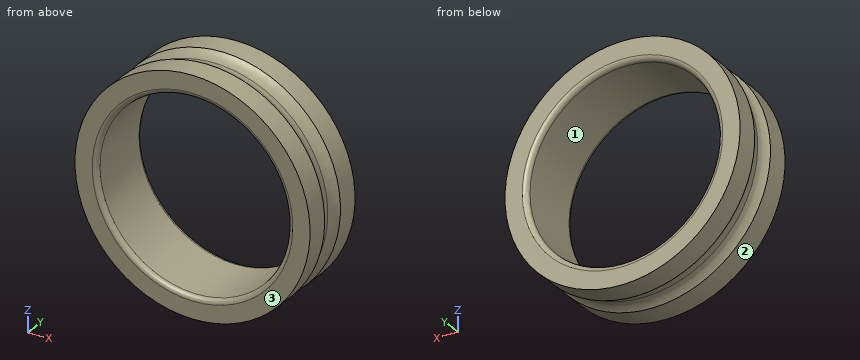
from build123d import *

# Parameters (mm, degrees)
FILLET1_R = 1


with BuildPart() as part:
    # Sketch1 → Revolve2 (revolve)
    with BuildSketch(Plane.XY, mode=Mode.PRIVATE) as revolve2_sk:
        with BuildLine():
            ThreePointArc((-23.61875, 7.5), (-23.878834577, 6.086926278), (-24.625, 4.859058821))
            Line((-24.625, 4.859058821), (-24.625, 0))
            Line((-24.625, 0), (-20, 0))
            Line((-20, 0), (-20, 15))
            Line((-20, 15), (-24.625, 15))
            Line((-24.625, 15), (-24.625, 10.140941179))
            ThreePointArc((-24.625, 10.140941179), (-23.878834577, 8.913073722), (-23.61875, 7.5))
        make_face()
    revolve(revolve2_sk.sketch.rotate(Axis((0, 0, 0), (0, 1, 0)), 270), axis=Axis((0, 0, 0), (0, 1, 0)))

    # Fillet1
    fillet1_edges = [part.edges().sort_by_distance(p)[0] for p in [
        (0, 15, 20),
        (0, 0, 20),
    ]]
    fillet(fillet1_edges, radius=FILLET1_R)


solid = part.part
The listing builds one solid part. Answer for the finished solid, in the listing's coordinates (mm). Face numbers are marked on the shaded views. Round coordinates to 2 decimals unless told otherwise and drop trailing zeros. Order: outer loops, then holes, each group sorted by start corner. A loop starts at its lowest first (then second) coordinate and runs counter-clockwise, first axis right, second up. Notation, with made-up numbers: (27, 48) -> (78, 48) arc R25 ccw to (78, 75) -> close; hole circle Ø7 at (75, 22.5). An arc over 180 degrees is marked (long way). One line per item, written item: value.
Item 1: Given P1, Ø1.5, axis at x = -17.5, y = 9, coming from the -Z side; P2, Ø6, axis at y = 10, z = 18, coming from the +X side; P3, Ø8, axis at x = -6, y = 8.5, coming from the -Z side, each flat-ended and moving along its own axis, determine where each tip first touches the part or whether it passes through.
Taken from the geometry:
P1: stops at z = -17.23
P2: stops at x = 19.53
P3: stops at z = -24.51
Item 2: Find section A-A, the plane y = 2.75. Give the vertices of the cut face in (x, z) (3 decimals), then the cut area to 3 significant figures.
Taken from the geometry:
outline: circle Ø49.25 at (0, 0); hole circle Ø40 at (0, 0)
area: 648 mm2
Item 3: Find section B-B, the plane y = 5.75. Give the vertices of the cut face in (x, z), then the cut area to 3 significant figures.
Taken from the geometry:
outline: circle Ø48.05 at (0, 0); hole circle Ø40 at (0, 0)
area: 557 mm2
Item 4: For a pull along Z with two mould halves and no side action, classify the marked faces 1, 2 and 3 as released by +Z, released by -Z, zero draft, split by the parting line, or undercut.
Taken from the geometry:
face 1: undercut
face 2: split by the parting line
face 3: zero draft
Item 5: Straight lines are drawn through the part: L1, parallel to X at y = 10.5, z = 0 (3 decimals); L2, parallel to Z at x = 2, y = 4.75; L3, parallel to Z at x = -16.5, y = 13.75. For each, find the intervals that lie inside material, in ascending order.
Taken from the geometry:
L1: x = -24.625 to -20, 20 to 24.625
L2: z = -24.54 to -19.9, 19.9 to 24.54
L3: z = -18.28 to -11.3, 11.3 to 18.28
